Job drawing, mm, ordinate dimensions from the low corner. One solid piece. A direction names the side the tool comes from. Coordinates: 2 decimals unless noted, no trailing zeros. Order: outer loops, then holes, each group sorted by start corner. A loop starts at its lowest first (then second) coordinate and runs counter-clockwise, first axis right, second up. Notation, with made-up numbers: (76.5, 66) -> (121.5, 66) arc R16 cw to (121.5, 96) -> close; hole circle Ø4 at (77.25, 75). An arc over 180 degrees is marked (long way). Use CSV: the item, a comma, the result in double quotes. Start each with the question number.
(1) Cut at D-D on y = 18.5. Write the cut outline in (x, z) (3 decimals).
(2) Tool access for the marked faces 1, 2, 3, 4 and 5: list every direction of +Z, -Z, +X, -X, +Y, -Y with a clear straight run to the whole face (end or side of a thin tool).
(3) Cut at B-B on z = 3.75. Write the cut outline in (x, y) (3 decimals).
(4) Cut at A-A on x = 20.5. Write the cut outline in (y, z) (3 decimals), plus the area to 3 significant figures.
(5) Probe L1, parallel to Y at x = 36, z = 4.5 (3 decimals); L2, parallel to X at y = 18, z = 1.5 (3 decimals); L3, parallel to X at y = 13, z = 14. List the from-to ranges inside material, lowest first.
(6) Pull direction Y, two halves, no side cores. Call the marked faces 6, 7 and 8: pulls with the +Y half, pulls with the -Y half, needs draft (parallel to the pull), parting line crosses it, or undercut.
(7) Pin check, flat tips, straight feed: pin 1 Ø4 at (x, z) = (24, 7.5) entering from +Y (3 decimals); pin 2 Ø10 at (y, z) = (20, 9) entering from +X; pin 3 Ø10 at (x, z) = (35.5, 3.5) entering from -Y (3 decimals); pin 4 Ø1.5 at (y, z) = (11.5, 11.5) entering from -X (3 decimals). Stop position of each tip, or through.
(8) Cut at C-C on y = 27.5. Write the cut outline in (x, z) (3 decimals).
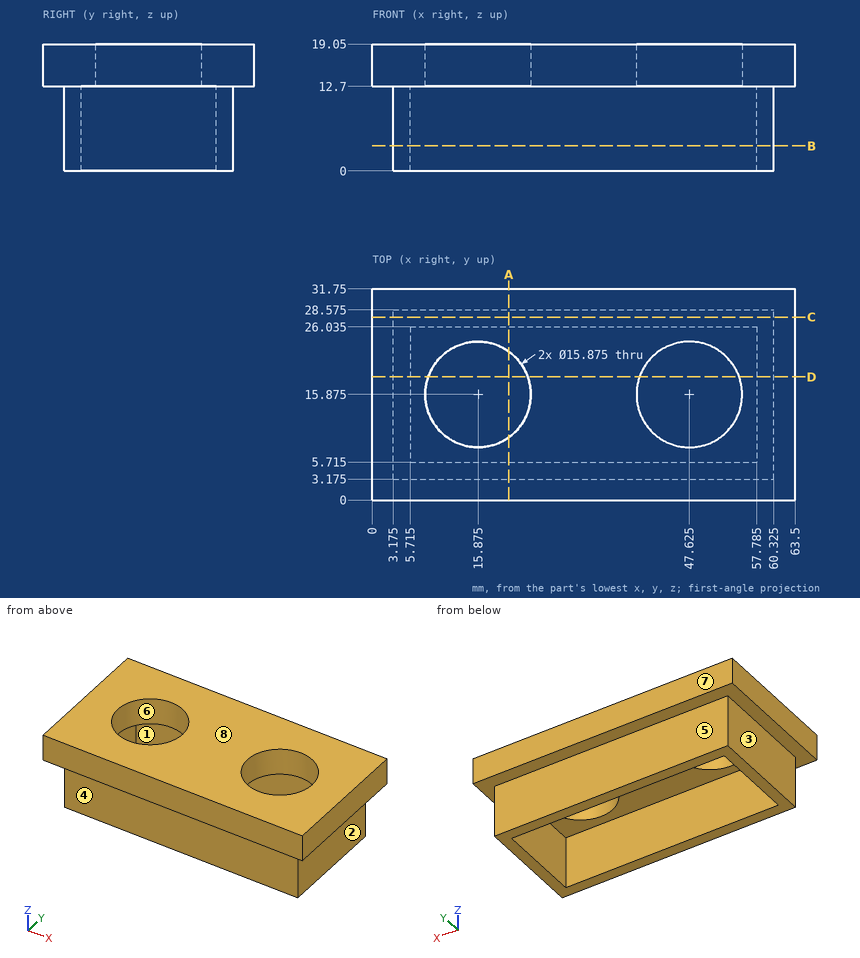
Outcome:
1,outline,"(0, 12.7) -> (3.175, 12.7) -> (3.175, 0) -> (5.715, 0) -> (5.715, 12.7) -> (8.384, 12.7) -> (8.384, 19.05) -> (0, 19.05) -> close; (23.366, 12.7) -> (40.134, 12.7) -> (40.134, 19.05) -> (23.366, 19.05) -> close; (55.116, 12.7) -> (57.785, 12.7) -> (57.785, 0) -> (60.325, 0) -> (60.325, 12.7) -> (63.5, 12.7) -> (63.5, 19.05) -> (55.116, 19.05) -> close"
2,face 1,"-Z"
2,face 2,"-Z, +X, +Y, -Y"
2,face 3,"-Z, -X, +Y, -Y"
2,face 4,"-Z, +X, -X, -Y"
2,face 5,"-Z, +X, -X, +Y"
3,outline,"(3.175, 3.175) -> (60.325, 3.175) -> (60.325, 28.575) -> (3.175, 28.575) -> close; hole (5.715, 5.715) -> (57.785, 5.715) -> (57.785, 26.035) -> (5.715, 26.035) -> close"
4,outline,"(0, 12.7) -> (3.175, 12.7) -> (3.175, 0) -> (5.715, 0) -> (5.715, 12.7) -> (9.424, 12.7) -> (9.424, 19.05) -> (0, 19.05) -> close; (22.326, 12.7) -> (26.035, 12.7) -> (26.035, 0) -> (28.575, 0) -> (28.575, 12.7) -> (31.75, 12.7) -> (31.75, 19.05) -> (22.326, 19.05) -> close"
4,area,"184 mm2"
5,L1,"3.175 to 5.715, 26.035 to 28.575"
5,L2,"3.175 to 5.715, 57.785 to 60.325"
5,L3,"0 to 8.48, 23.27 to 40.23, 55.02 to 63.5"
6,face 6,"undercut"
6,face 7,"pulls with the +Y half"
6,face 8,"needs draft"
7,pin 1,"y = 28.575"
7,pin 2,"x = 63.5"
7,pin 3,"y = 3.175"
7,pin 4,"x = 3.175"
8,outline,"(0, 12.7) -> (3.175, 12.7) -> (3.175, 0) -> (60.325, 0) -> (60.325, 12.7) -> (63.5, 12.7) -> (63.5, 19.05) -> (0, 19.05) -> close"
